The listing builds one solid part. Answer for the finished solid, in the listing's coordinates (mm). Face numbers are marked on the shaded views. Round coordinates to 2 decimals unless told otherwise and drop trailing zeros. Write each loop counter-clockwise with the first axis right and the second up, starting at its lowest first coordinate (ties: lowest second). Pieces come first, ordered by that corner, then holes.
Item 1: Find section A-A on x = 0. Give the vertices of the cut face in (y, z).
Item 2: Find section D-D on x = 11.5. Give the vertices of the cut face in (y, z), then the cut area to 3 significant figures.
Item 3: Each of these flat-tipped pins is pushed along its axis until it touches: pin 1 (16.5 mm diameter, centred on x = 0, z = 0, fed in from -Y); pin 2 (1.5 mm diameter, centred on y = 15, z = -8.5, fed in from +X); pin 3 (5 mm diameter, centred on y = 14.5, z = -2.5, fed in from -X); pin 4 (1.5 mm diameter, centred on x = -11, y = 16, fed in from +Z). Where does it stop, or does it pass through?
Item 4: Find section B-B on z = 0. Give the vertices of the cut face in (x, y), then the cut area to 3 significant figures.
Item 5: Find the intervals of material crossed by probe 1 along Z at (x, y) = (0, 17.5); probe 2 along X at (y, z) = (7.25, 4); probe 3 along X at (y, z) = (20.75, 6.5), in increasing order.
Item 6: Find section C-C on y = 4. Give the vertices of the cut face in (x, z), then the cut area to 3 significant figures.
Item 7: For a pull along X with two mould halves and no side action, classify the marked faces 1, 2 and 3 as +X half, -X half, draft (parallel to the pull), parting line (faces both ways), or undercut.
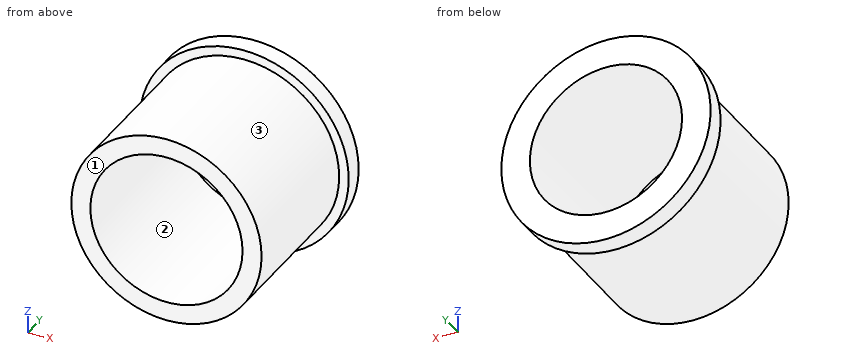
```python
from build123d import *

# Parameters (mm, degrees)
SKETCH1_R           = 12.7
BOSS_EXTRUDE1_DEPTH = 19.812
SKETCH2_R           = 13.97
BOSS_EXTRUDE2_DEPTH = 2.54
SKETCH3_R           = 10.16
CUT_EXTRUDE1_DEPTH  = 23.352


with BuildPart() as part:
    # Sketch1 → Boss-Extrude1 (new body)
    with BuildSketch(Plane(origin=(0, 0, 0), x_dir=(1, 0, 0), z_dir=(0, 1, 0))):
        Circle(SKETCH1_R)
    extrude(amount=BOSS_EXTRUDE1_DEPTH)

    # Sketch2 → Boss-Extrude2 (add)
    with BuildSketch(Plane(origin=(0, 19.812, 0), x_dir=(1, 0, 0), z_dir=(0, 1, 0))):
        Circle(SKETCH2_R)
    extrude(amount=BOSS_EXTRUDE2_DEPTH)

    # Sketch3 → Cut-Extrude1 (cut, through all)
    with BuildSketch(Plane.XZ):
        Circle(SKETCH3_R)
    extrude(amount=-CUT_EXTRUDE1_DEPTH, mode=Mode.SUBTRACT)


solid = part.part
```
Check values:
1. outline: (0, -12.7) - (19.81, -12.7) - (19.81, -13.97) - (22.35, -13.97) - (22.35, -10.16) - (0, -10.16) - close; (0, 10.16) - (22.35, 10.16) - (22.35, 13.97) - (19.81, 13.97) - (19.81, 12.7) - (0, 12.7) - close
2. outline: (0, -5.39) - (19.81, -5.39) - (19.81, -7.93) - (22.35, -7.93) - (22.35, 7.93) - (19.81, 7.93) - (19.81, 5.39) - (0, 5.39) - close
2. area: 254 mm2
3. pin 1: passes through
3. pin 2: stops at x = 10.06
3. pin 3: stops at x = -12.7
3. pin 4: stops at z = 7.5
4. outline: (-13.97, 19.81) - (-12.7, 19.81) - (-12.7, 0) - (-10.16, 0) - (-10.16, 22.35) - (-13.97, 22.35) - close; (10.16, 0) - (12.7, 0) - (12.7, 19.81) - (13.97, 19.81) - (13.97, 22.35) - (10.16, 22.35) - close
4. area: 120 mm2
5. probe 1: z = -12.7 to -10.16, 10.16 to 12.7
5. probe 2: x = -12.05 to -9.34, 9.34 to 12.05
5. probe 3: x = -12.37 to -7.81, 7.81 to 12.37
6. outline: circle Ø25.4 at (0, 0); hole circle Ø20.32 at (0, 0)
6. area: 182 mm2
7. face 1: draft
7. face 2: undercut
7. face 3: parting line
